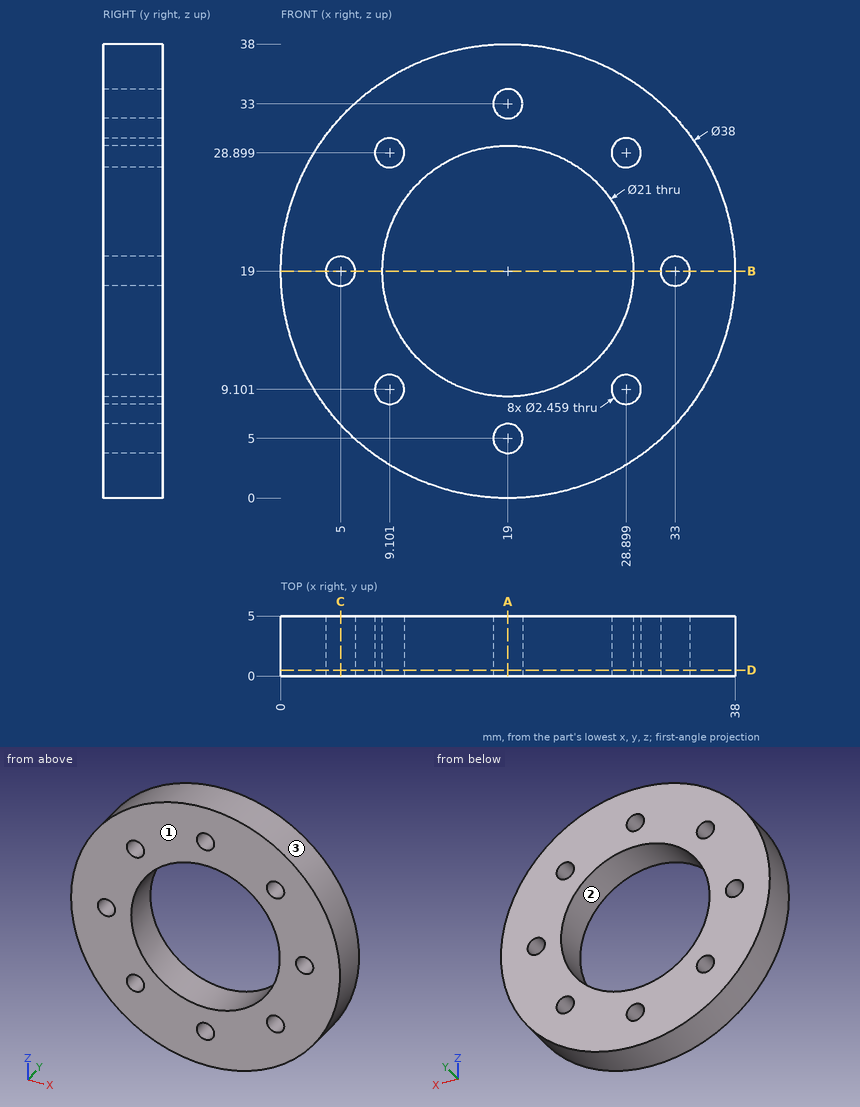
Here's the drawing with two shaded views (mm, measured from the low corner). I have some questions. Round coordinates to 2 decimals unless told otherwise and drop trailing zeros. Loops run counter-clockwise (first coordinate to the right, second up) from the corner with the lowest first, then second, coordinate; pieces in that order, holes last. Notation, with made-up numbers: M -21,10 L -10,10 A23 cw -10,35 Z; hole C 15.5,-9.5 d2. An arc over 180 degrees is marked long. Put each result on its own line as item: value.
Q1. Thinking about a two-plate mould opening in X: for the marked faces 1, 2 and 3, which applies, released by +X, released by -X, zero draft, split by the parting line, or undercut?
Check result:
face 1: zero draft
face 2: undercut
face 3: split by the parting line
Q2. Imagine slicing it at C-C (x = 5). Write out the boundary of the cut face in (y, z) (1 decimal), then the cut area to 3 significant figures.
Check result:
outline: M 0,6.2 L 5,6.2 L 5,17.8 L 0,17.8 Z; M 0,20.2 L 5,20.2 L 5,31.8 L 0,31.8 Z
area: 116 mm2
Q3. Imagine slicing it at B-B (z = 19). Write out the boundary of the cut face in (x, y).
Check result:
outline: M 0,0 L 3.77,0 L 3.77,5 L 0,5 Z; M 6.23,0 L 8.5,0 L 8.5,5 L 6.23,5 Z; M 29.5,0 L 31.77,0 L 31.77,5 L 29.5,5 Z; M 34.23,0 L 38,0 L 38,5 L 34.23,5 Z
Q4. I need wall thicknesses on probe 1 along Z at (x, y) = (19, 1.1); probe 2 along Z at (x, y) = (12.5, 0.9) (1 decimal); probe 3 along Z at (x, y) = (22, 0.35). Which ranges of each line are inside material? Lowest first, please.
Check result:
probe 1: 0 to 3.77, 6.23 to 8.5, 29.5 to 31.77, 34.23 to 38
probe 2: 1.1 to 10.8, 27.2 to 36.9
probe 3: 0.24 to 8.94, 29.06 to 37.76
Q5. For pin 1 (2 mm diameter, centred on x = 28.9, z = 28.9, fed in from +Y); pin 2 (1.5 mm diameter, centred on y = 4.5, z = 14, fed in from +X); pin 3 (1 mm diameter, centred on x = 15.5, y = 4, fed in from -Z), each with a flat end and sliding along its axis, tell me the tip position at first contact or that it passes through.
Check result:
pin 1: through
pin 2: x = 37.52
pin 3: z = 0.24
Q6. Imagine slicing it at D-D (y = 0.5). State how many separate pieces and enclosed holes the cut face has, then the cut area to 3 significant figures.
Check result:
separate pieces: 1
enclosed holes: 9
area: 750 mm2
Q7. Imagine slicing it at A-A (x = 19). Write out the boundary of the cut face in (y, z).
Check result:
outline: M 0,0 L 5,0 L 5,3.77 L 0,3.77 Z; M 0,6.23 L 5,6.23 L 5,8.5 L 0,8.5 Z; M 0,29.5 L 5,29.5 L 5,31.77 L 0,31.77 Z; M 0,34.23 L 5,34.23 L 5,38 L 0,38 Z
